Work out the finished part from the listing and answer in its coordinate system (mm). Face numbers are marked on the shaded views. A direction names the side the tool comes from. Round coordinates to 2 decimals unless told otherwise and drop trailing zeros. Order: outer loops, then holes, each group sorted by start corner. A loop starts at its lowest first (then second) coordinate and runs counter-clockwise, first axis right, second up. Notation, with made-up numbers: (61, -23) - (70, -23) arc R18 ccw to (70, -7) - close; hole circle Ø4 at (28.5, 23). An arc over 180 degrees is marked (long way). Answer in a Markdown table with one row per item.
Autodesk Inventor part; units mm, degrees
ref_plane "YZ Plane" through (0, 0, 0) normal (1, 0, 0) x (0, 1, 0)
ref_plane "XZ Plane" through (0, 0, 0) normal (0, 1, 0) x (-1, 0, 0)
ref_plane "XY Plane" through (0, 0, 0) normal (0, 0, 1) x (1, 0, 0)
sketch "Sketch1" plane through (0, 0, 0) normal (0, 0, 1) x (1, 0, 0)
  line L0 (0, 0) -> (-90, 0)
  line L1 (-90, 0) -> (-90, -1490)
  line L2 (-90, -1490) -> (0, -1490)
  line L3 (0, -1490) -> (0, 0)
  line L4 (-90, -1390) -> (-40, -1390)
  line L5 (-40, -1390) -> (-40, -1385)
  line L6 (-40, -1385) -> (-90, -1385)
  line L7 (-90, -1385) -> (-90, -1390)
  line L8 (-90, -893.3333) -> (-40, -893.3333)
  line L9 (-40, -893.3333) -> (-40, -888.3333)
  line L10 (-40, -888.3333) -> (-90, -888.3333)
  line L11 (-90, -888.3333) -> (-90, -893.3333)
  line L12 (-90, -396.6667) -> (-40, -396.6667)
  line L13 (-40, -396.6667) -> (-40, -391.6667)
  line L14 (-40, -391.6667) -> (-90, -391.6667)
  line L15 (-90, -391.6667) -> (-90, -396.6667)
  circle A0 centre (-90, -155) radius 30
  line L16 (-90, -155) -> (0, -155)
  line L17 (-90, -953) -> (0, -953)
  point P0 (-90, -391.6667)
  point P1 (-90, -396.6667)
  point P2 (-90, -888.3333)
  point P3 (-90, -893.3333)
  point P4 (-90, -125)
  point P5 (-90, -185)
  point P6 (-60, -155)
  dimension "d0" = 1490
  dimension "d1" = 90
  dimension "d2" = 5
  dimension "d4" = 100
  dimension "d7" = 496.6667
  dimension "d23" = 40
  dimension "d28" = 60
  dimension "d30" = 1335
  dimension "d31" = 953
extrude "Plate1" add sketch "Sketch1" along normal blind 4 contours L3 L17 L1 L8 L9 L10 L12 L13 L14 A0 L16
sketch "Sketch2" plane through (-4, -155, 0) normal (1, 0, 0) x (0, 1, 0)
  line L0 (-798, 0) -> (0, 0)
  line L1 (0, 0) -> (0, 60)
  line L2 (0, 60) -> (-798, 60)
  line L3 (-798, 60) -> (-798, 0)
edge flange "Flange1" height 60 angle 90 thickness 4 bend radius 4 thickness toward (1, 0, 0) relief tear relief width 4 relief depth 2 edges at (0, -554, 4) wall of the first edge with corners at (-4, -953, 0) (-4, -155, 0) (-4, -155, 60) (-4, -953, 60)
bend "Bend1"
corner "Corner1"
chamfer "Corner Chamfer1" distance 3 angle 45 4 edges at (-90, -893.3333, 2) (-90, -888.3333, 2) (-90, -391.6667, 2) (-90, -396.6667, 2)
equation "\"d0\" = Стрингер_длина"
equation "\"d2\" = паз_под_стрингер_толщина"
equation "\"d7\" = Шаг_шпангоутов"
equation "\"d28\" = 2 * радиус_выреза_под_сварку"
equation "\"d12\" = Thickness"
equation "\"d13\" = BendReliefWidth"
equation "\"d14\" = BendReliefDepth"
equation "\"d15\" = MinimumRemnant"
equation "\"d16\" = TransitionRadius"
equation "\"d17\" = ребро_усилителей"
equation "\"d19\" = BendRadius"
equation "\"d20\" = CornerReliefSize"
equation "\"d21\" = GapSize"
equation "\"d22\" = JacobiRadiusSize"
equation "\"BendRadius\" = Thickness"
equation "\"BendReliefWidth\" = Thickness"
equation "\"BendReliefDepth\" = 0.5 * Thickness"
equation "\"CornerReliefSize\" = 4 * Thickness"
equation "\"MinimumRemnant\" = 2 * Thickness"
equation "\"TransitionRadius\" = BendRadius"
equation "\"JacobiRadiusSize\" = BendRadius"
equation "\"GapSize\" = Thickness"
properties part number "GBK 0103 stringer 2_Dummy" material "Steel"
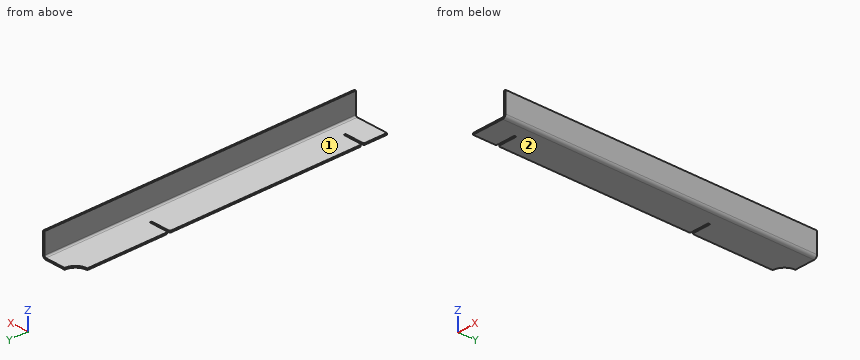
1) Find section C-C, the plane z = 32.5. Give the vertices of the cut face in (x, y).
Filled in:
| item | result |
|---|---|
| outline | (-4, -953) - (0, -953) - (0, -155) - (-4, -155) - close |
2) Which of the six approach directions +Z, -Z, +X, -X, +Y, -Y give full straight-line access (tool end or side, diameter ignored) to the marked faces 1 and 2?
Filled in:
| item | result |
|---|---|
| face 1 | +Z, -X, +Y, -Y |
| face 2 | -Z, +X, -X, +Y, -Y |
3) Each of these flat-tipped pins is pushed along its axis until it touches: pin 1 (1.2 mm diameter, centred on y = -889.5, z = 1.5, fed in from -X); pin 2 (1.5 mm diameter, centred on x = -59.5, y = -852, fed in from +Z); pin 3 (15.5 mm diameter, centred on y = -488.5, z = 22.5, fed in from -X). Where does it stop, or does it pass through?
Filled in:
| item | result |
|---|---|
| pin 1 | stops at x = -40 |
| pin 2 | stops at z = 4 |
| pin 3 | stops at x = -4 |
4) Find section D-D, the plane x = -22. Give the vertices of the cut face in (y, z).
Filled in:
| item | result |
|---|---|
| outline | (-953, 0) - (-155, 0) - (-155, 4) - (-953, 4) - close |
5) Find the intervals of material crossed by probe 1 along Z at (x, y) = (-66.5, -319); probe 2 along X at (y, z) = (-338, 56); probe 3 along Z at (x, y) = (-7, -518), in increasing order. Write a range as from..to.
Filled in:
| item | result |
|---|---|
| probe 1 | z = 0..4 |
| probe 2 | x = -4..0 |
| probe 3 | z = 0.06..4.13 |
6) Find section A-A, the plane x = -73. Give the vertices of the cut face in (y, z).
Filled in:
| item | result |
|---|---|
| outline | (-953, 0) - (-893.33, 0) - (-893.33, 4) - (-953, 4) - close; (-888.33, 0) - (-396.67, 0) - (-396.67, 4) - (-888.33, 4) - close; (-391.67, 0) - (-179.72, 0) - (-179.72, 4) - (-391.67, 4) - close |
7) Find section B-B, the plane y = -758. Give the vertices of the cut face in (x, z).
Filled in:
| item | result |
|---|---|
| outline | (-90, 0) - (-8, 0) arc R8 ccw to (0, 8) - (0, 60) - (-4, 60) - (-4, 8) arc R4 cw to (-8, 4) - (-90, 4) - close |
